```python
from build123d import *

# Parameters (mm, degrees)
F0_R     = 2.5
F1_DEPTH = 4


with BuildPart() as f1:
    # F0 (on Top) → F1 (new body)
    with BuildSketch(Plane.XY):
        with BuildLine():
            Line((-12.856996, -12.678498), (12.856996, -12.678498))
            ThreePointArc((12.856996, -12.678498), (34.195831, -21.517333), (25.356996, -0.178498))
            Line((25.356996, -0.178498), (25.356996, 0.178498))
            ThreePointArc((25.356996, 0.178498), (34.195831, 21.517333), (12.856996, 12.678498))
            Line((12.856996, 12.678498), (5, 12.678498))
            ThreePointArc((5, 12.678498), (0, 17.678498), (-5, 12.678498))
            Line((-5, 12.678498), (-12.856996, 12.678498))
            ThreePointArc((-12.856996, 12.678498), (-34.195831, 21.517333), (-25.356996, 0.178498))
            Line((-25.356996, 0.178498), (-25.356996, -0.178498))
            ThreePointArc((-25.356996, -0.178498), (-34.195831, -21.517333), (-12.856996, -12.678498))
        make_face()
        with Locations((0, 12.678498)):
            Circle(F0_R, mode=Mode.SUBTRACT)
    extrude(amount=F1_DEPTH)


solid = f1.part
```
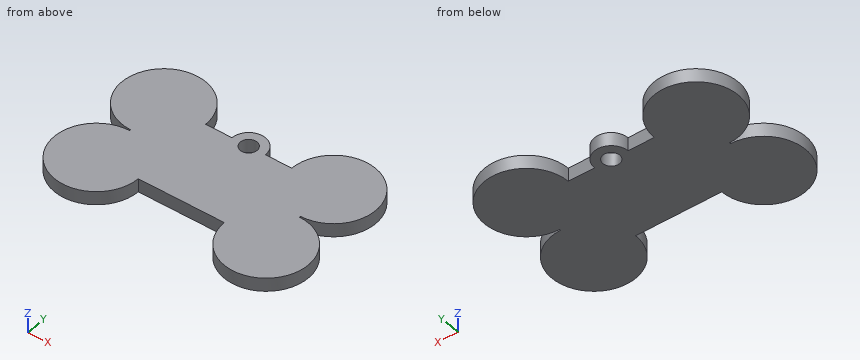
Geometry check sheet. Reference: the model listing, model coordinates, mm. Give positions to 0.01 mm unless a question says otherwise; leave off trailing zeros. Loops run counter-clockwise (first coordinate to the right, second up) from the corner with the lowest first, then second, coordinate; pieces in that order, holes last. Notation, with made-up numbers: M 79.25,-1 L 99.25,-1 A19 cw 99.25,10 Z; hole C -40,-22.5 d8. An arc over 180 degrees is marked long. Write item = value, one per line. Start each with the question number.
1. Section check D-D, the plane y = -14. Enter the section's corners in (x, z), plus the area to 3 significant figures.
2. Section check C-C, the plane y = 16. Enter the section's corners in (x, z).
3. Go/stop test with flat-tipped pins: P1, Ø1.2, axis at x = -10, z = 1.5, coming from the +Y side; P2, Ø1.5, axis at y = 20, z = 2.5, coming from the -X side; P3, Ø2, axis at x = -28.5, z = 0.5, coming from the -Y side. Record where each tip stops, or that it passes through.
4. Section check A-A, the plane x = 0. Enter the section's corners in (y, z), plus the area to 3 significant figures.
5. Thickness scan on probe 1 along Y at (x, z) = (0, 1.9); probe 2 along Y at (x, z) = (26, 3.4); probe 3 along X at (y, z) = (-19, 2.4). Record the ranges inside material, lowest first.
6. Section check B-B, the plane z = 1.15. Enter the section's corners in (x, y).
Values follow:
q1.outline = M -37.79,0 L -12.93,0 L -12.93,4 L -37.79,4 Z; M 12.93,0 L 37.79,0 L 37.79,4 L 12.93,4 Z
q1.area = 199 mm^2
q2.outline = M -37.41,0 L -13.31,0 L -13.31,4 L -37.41,4 Z; M -3.74,0 L 3.74,0 L 3.74,4 L -3.74,4 Z; M 13.31,0 L 37.41,0 L 37.41,4 L 13.31,4 Z
q3.P1 = 12.68
q3.P2 = -35.99
q3.P3 = -24.99
q4.outline = M -12.68,0 L 10.18,0 L 10.18,4 L -12.68,4 Z; M 15.18,0 L 17.68,0 L 17.68,4 L 15.18,4 Z
q4.area = 101 mm^2
q5.probe_1 = -12.68 to 10.18, 15.18 to 17.68
q5.probe_2 = -25.16 to -0.2, 0.2 to 25.16
q5.probe_3 = -36.14 to -14.57, 14.57 to 36.14
q6.outline = M -25.36,-0.18 A12.5 ccw long -12.86,-12.68 L 12.86,-12.68 A12.5 ccw long 25.36,-0.18 L 25.36,0.18 A12.5 ccw long 12.86,12.68 L 5,12.68 A5 ccw -5,12.68 L -12.86,12.68 A12.5 ccw long -25.36,0.18 Z; hole C 0,12.68 d5
